from build123d import *

# Parameters (mm, degrees)
BOSS_EXTRUDE1_START = 66.421062
BOSS_EXTRUDE1_DEPTH = 3.175
FILLET1_R           = 9.525


with BuildPart() as part:
    # Sketch1 → Boss-Extrude1 (new body)
    with BuildSketch(Plane(origin=(0, 0, 0), x_dir=(0, 0, -1), z_dir=(1, 0, 0)).offset(BOSS_EXTRUDE1_START)):
        with BuildLine():
            Line((-1321.232047874, 253.01907305), (-1270.768280058, 312.11266745))
            ThreePointArc((-1270.768280058, 312.11266745), (-1269.714759772, 322.976697122), (-1279.556254241, 327.697081886))
            Line((-1279.556254241, 327.697081886), (-1304.620022056, 323.577914146))
            ThreePointArc((-1304.620022056, 323.577914146), (-1310.336145998, 320.343921033), (-1312.600334154, 314.179001215))
            Line((-1312.600334154, 314.179001215), (-1312.600334154, 294.129574554))
            Line((-1312.600334154, 294.129574554), (-1328.475334154, 294.129574554))
            ThreePointArc((-1328.475334154, 294.129574554), (-1335.210526245, 291.339766645), (-1338.000334154, 284.604574554))
            Line((-1338.000334154, 284.604574554), (-1338.000334154, 259.204574554))
            ThreePointArc((-1338.000334154, 259.204574554), (-1331.771796135, 250.268190307), (-1321.232047874, 253.01907305))
        make_face()
    extrude(amount=BOSS_EXTRUDE1_DEPTH)

    # Fillet1
    fillet1_edges = [part.edges().sort_by_distance(p)[0] for p in [
        (68.008562, 294.129574554, 1312.600334154),
    ]]
    fillet(fillet1_edges, radius=FILLET1_R)


solid = part.part
Work out the finished part from the listing and answer in its coordinate system (mm). A direction names the side the tool comes from. Give positions to 0.01 mm unless a question says otherwise; leave off trailing zeros. Write each loop counter-clockwise with the first axis right and the second up, starting at its lowest first coordinate (ties: lowest second). Pieces come first, ordered by that corner, then holes. Notation, with made-up numbers: (-37, 37.5) - (-17, 37.5) arc R13 ccw to (-17, 58.5) - close; hole circle Ø7 at (-34, 34). An arc over 180 degrees is marked (long way). One line per item, written item: value. Start each with the question number.
1. Given pin 1 (1.5 mm diameter, centred on x = 67.5, y = 306.5, fed in from -Z), flat-ended and moving along its own axis, determine where the tip first touches the part or whether it passes through.
2. Consider probe 1 along Y at (x, z) = (68, 1283); probe 2 along Y at (x, z) = (68.5, 1317.5); probe 3 along Z at (x, y) = (68.25, 286). Determine where each line is inside the solid, lowest interval first.
3. Find section A-A (x = 67.8). Write down the section's boundary in (y, z) (3 decimals), then the cut area to 3 significant figures.
4. For faces 1 (the flat face through (68, 294.13, 1325)), 2 (the cylindrical face through (67.986, 250.326, 1331.924)), determine the directions among +Z, -Z, +X, -X, +Y, -Y from which every point of the face is accessible in a straight line to the end or side of a thin tool.
5. Find section B-B (y = 304.5). Write down the section's boundary in (x, z), then the cut area to 3 significant figures.
6. Find section C-C (z = 1325.5). Write down the section's boundary in (x, y), then the cut area to 3 significant figures.
Geometry results:
1. pin 1: z = 1274.92
2. probe 1: 297.79 to 327.13
2. probe 2: 257.39 to 295.33
2. probe 3: 1293.07 to 1337.9
3. outline: (253.019, 1321.232) - (312.113, 1270.768) arc R9.525 ccw to (327.697, 1279.556) - (323.578, 1304.62) arc R9.525 ccw to (314.179, 1312.6) - (303.655, 1312.6) arc R9.525 cw to (294.13, 1322.125) - (294.13, 1328.475) arc R9.525 ccw to (284.605, 1338) - (259.205, 1338) arc R9.525 ccw to start
3. area: 2,620 mm2
4. face 1: +Z, +X, -X, +Y
4. face 2: +X, -X, -Y
5. outline: (66.42, 1277.27) - (69.6, 1277.27) - (69.6, 1312.6) - (66.42, 1312.6) - close
5. area: 112 mm2
6. outline: (66.42, 250.16) - (69.6, 250.16) - (69.6, 294.13) - (66.42, 294.13) - close
6. area: 140 mm2
